Geometry: see drawing. Coordinates: mm, zero at the bounding-box minimum. Coordinates: 2 decimals unless noted, no trailing zeros. Order: outer loops, then holes, each group sorted by start corner. A loop starts at its lowest first (then second) coordinate and runs counter-clockwise, first axis right, second up. Notation, with made-up numbers: (77.25, 10.25) -> (106.25, 10.25) arc R36 ccw to (106.25, 47.25) -> close; hole circle Ø10 at (30, -1.75). An arc over 180 degrees is marked (long way). Write each question's results on one line, items separated by ' | '.
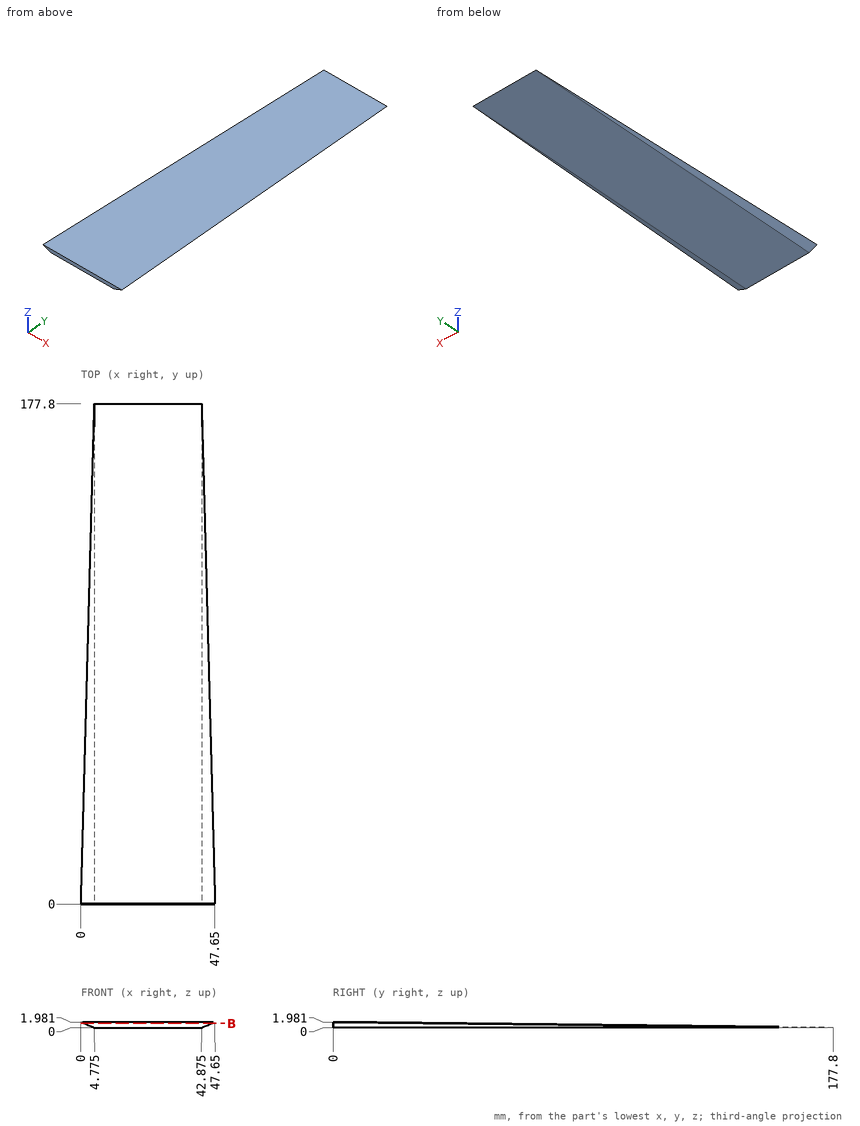
(1) Line query: line 1 along X through (y, z) = (144.5, 0.15) (1 decimal); line 2 along X through (y, z) = (52.5, 1.1) (1 decimal); line 3 along Z through (x, y) = (45, 84.5). Output: solid intervals per line, ascending. Write a range as from..to.
Return value:
line 1: 4.4..43.2 | line 2: 2.1..45.5 | line 3: 0.88..1.04
(2) Cut plane B-B, the plane z = 1.5. Return loops of the section in (x, y) (1 decimal), plus the area to 3 significant figures.
Return value:
outline: (1.2, 0) -> (46.5, 0) -> (46.5, 43.2) -> (1.2, 43.2) -> close | area: 1,960 mm2
(3) Pin query (flat end, axial travel): P1, Ø1, axis at y = 115.5, z = 0.5, coming from the +X side; P2, Ø2, axis at x = 37.5, y = 24.5, coming from the +Z side. Return the tip coordinate at first contact, or that it passes through.
Return value:
P1: x = 44.56 | P2: z = 1.72
